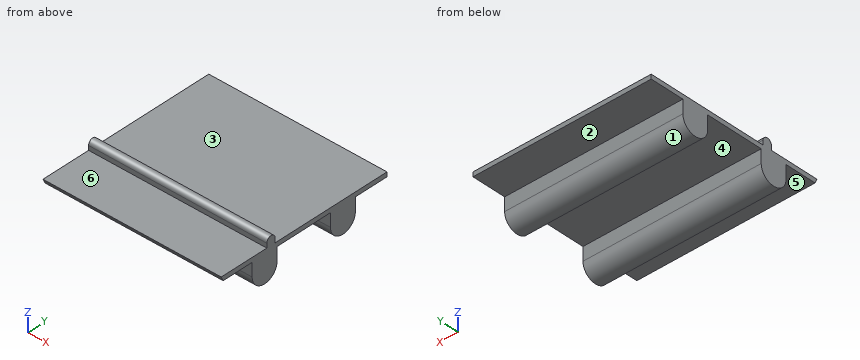
```python
from build123d import *

# Parameters (mm, degrees)
SKETCH1_W           = 127
SKETCH1_H           = 127
BOSS_EXTRUDE1_DEPTH = 3.175
CUT_EXTRUDE1_DEPTH  = 143.025809714
BOSS_EXTRUDE3_DEPTH = 127
BOSS_EXTRUDE4_DEPTH = 127


with BuildPart() as part:
    # Sketch1 → Boss-Extrude1 (new body)
    with BuildSketch(Plane.XY):
        Rectangle(SKETCH1_W, SKETCH1_H)
    extrude(amount=BOSS_EXTRUDE1_DEPTH)

    # Sketch2 → Cut-Extrude1 (cut, through all)
    with BuildSketch(Plane(origin=(63.5, 0, 0), x_dir=(0, 0, -1), z_dir=(1, 0, 0))):
        Polygon((-3.175, -63.5), (0, -62.019473185), (0, -63.5), align=None)
    extrude(amount=-CUT_EXTRUDE1_DEPTH, mode=Mode.SUBTRACT)

    # Sketch3 → Boss-Extrude3 (add)
    with BuildSketch(Plane(origin=(63.5, 0, 0), x_dir=(0, 0, -1), z_dir=(1, 0, 0))):
        with BuildLine():
            Line((9.525, 39.255526815), (0, 39.255526815))
            Line((0, 39.255526815), (0, 20.205526815))
            Line((0, 20.205526815), (9.525, 20.205526815))
            ThreePointArc((9.525, 20.205526815), (19.05, 29.730526815), (9.525, 39.255526815))
        make_face()
        with BuildLine():
            Line((9.525, -20.744473185), (0, -20.744473185))
            Line((0, -20.744473185), (0, -39.794473185))
            Line((0, -39.794473185), (9.525, -39.794473185))
            ThreePointArc((9.525, -39.794473185), (19.05, -30.269473185), (9.525, -20.744473185))
        make_face()
    extrude(amount=-BOSS_EXTRUDE3_DEPTH)

    # Sketch4 → Boss-Extrude4 (add)
    with BuildSketch(Plane(origin=(63.5, 0, 0), x_dir=(0, 0, -1), z_dir=(1, 0, 0))):
        with BuildLine():
            Line((-6.35, -22.225), (-3.175, -22.225))
            Line((-3.175, -22.225), (-3.175, -28.575))
            Line((-3.175, -28.575), (-6.35, -28.575))
            ThreePointArc((-6.35, -28.575), (-9.525, -25.4), (-6.35, -22.225))
        make_face()
    extrude(amount=-BOSS_EXTRUDE4_DEPTH)


solid = part.part
```
For this review, take the finished solid that the model builds, in its own axes (mm). Face numbers are marked on the shaded views. A direction names the side the tool comes from. Round coordinates to 2 decimals unless told otherwise and drop trailing zeros. Loops run counter-clockwise (first coordinate to the right, second up) from the corner with the lowest first, then second, coordinate; pieces in that order, holes last.
(1) We need section C-C (y = -55.5). Give the boundary of the cut face in (x, z) (3 decimals), plus the area to 3 significant figures.
Returned:
outline: (-63.5, 0) - (63.5, 0) - (63.5, 3.175) - (-63.5, 3.175) - close
area: 403 mm2
(2) We need section D-D (y = -25.4). Give the boundary of the cut face in (x, z) (3 decimals).
Returned:
outline: (-63.5, -17.711) - (63.5, -17.711) - (63.5, 9.525) - (-63.5, 9.525) - close
(3) Mouldability with a two-part tool opening along Y and no side actions: class the marked faces 1 and 2 as released by +Y, released by -Y, zero draft, split by the parting line, or undercut.
Returned:
face 1: undercut
face 2: zero draft
(4) We need section A-A (x = -5). Give the boundary of the cut face in (y, z) (3 decimals), plus the area to 3 significant figures.
Returned:
outline: (-63.5, 3.175) - (-62.019, 0) - (-39.794, 0) - (-39.794, -9.525) arc R9.525 ccw to (-20.744, -9.525) - (-20.744, 0) - (20.206, 0) - (20.206, -9.525) arc R9.525 ccw to (39.256, -9.525) - (39.256, 0) - (63.5, 0) - (63.5, 3.175) - (-22.225, 3.175) - (-22.225, 6.35) arc R3.175 ccw to (-28.575, 6.35) - (-28.575, 3.175) - close
area: 1,080 mm2
(5) We need section B-B (z = -16.25). Give the boundary of the cut face in (x, y), plus the area to 3 significant figures.
Returned:
outline: (-63.5, -37.01) - (63.5, -37.01) - (63.5, -23.52) - (-63.5, -23.52) - close; (-63.5, 22.99) - (63.5, 22.99) - (63.5, 36.48) - (-63.5, 36.48) - close
area: 3,430 mm2
(6) Tool access review of the marked faces 3, 4, 5 and 6: name each direction out of +Z, -Z, +X, -X, +Y, -Y from which nothing blocks a thin tool from reaching the whole face with its end or side.
Returned:
face 3: +Z, +X, -X, +Y
face 4: -Z, +X, -X
face 5: -Z, +X, -X, -Y
face 6: +Z, +X, -X, -Y
(7) Wall thickness on line 1 along Y through (x, z) = (29.5, -0.75); line 2 along Z through (x, y) = (-42.5, 48.5) (3 decimals); line 3 along Y through (x, z) = (-25.5, -12.75): over which ranges is each line inside the solid? List them lowest first.
Returned:
line 1: y = -39.79 to -20.74, 20.21 to 39.26
line 2: z = 0 to 3.175
line 3: y = -39.23 to -21.31, 20.77 to 38.69
(8) Clearance check with flat-ended pins moving along their axes: P1, Ø5, axis at x = -17.5, z = -6, coming from the +Y side; P2, Ø7.5, axis at x = 31.5, z = -4.5, coming from the -Y side; P3, Ø4, axis at x = 22.5, y = 47, coming from the +Z side (3 decimals). State where each tip first meets the part, or that it passes through.
Returned:
P1: stops at y = 39.26
P2: stops at y = -39.79
P3: stops at z = 3.175
